Input: part model. Units: mm. Frame: model coordinates. Face numbers are marked on the shaded views. A direction names the side the tool comes from. Round coordinates to 2 decimals unless told otherwise and drop trailing zeros. Loops run counter-clockwise (first coordinate to the right, second up) from the corner with the lowest first, then second, coordinate; pieces in that order, holes last.
1) Access query for the marked faces 4 and 5. Directions: +Z, -Z, +X, -X, +Y, -Y. A direction counts if a zero-diameter tool reaches every point of the face in a straight line with its end or side. Return the directions, or none.
2) Draft query along Y for the marked faces 1, 2 and 3. Return one class per face: pulls with the +Y half, pulls with the -Y half, needs draft (parallel to the pull), parting line crosses it, or undercut.
3) Section A-A, the plane x = 0. Return loops of the section in (y, z), and give its area (3 significant figures).
4) Section D-D, the plane z = 4.5. Return loops of the section in (x, y).
5) Ray query, line 1 along Z through (x, y) = (4.75, 1.5); line 2 along Y through (x, z) = (0, 6.75); line 3 along X through (y, z) = (1.25, 7). Return the intervals inside material, ascending.
6) Section C-C, the plane y = -2.5. Return loops of the section in (x, z).
7) First-contact query: pin 1 (3 mm diameter, centred on x = -1.5, z = 3.5, fed in from -Y); pin 2 (1.5 mm diameter, centred on x = -3.5, z = 4.5, fed in from -Y); pin 3 (1.5 mm diameter, centred on x = -3.5, z = 2.5, fed in from +Y); pin 4 (1.8 mm diameter, centred on x = 0, y = 0, fed in from -Z). Flat tips, straight axial feed; report the tip coordinate or a pass-through.
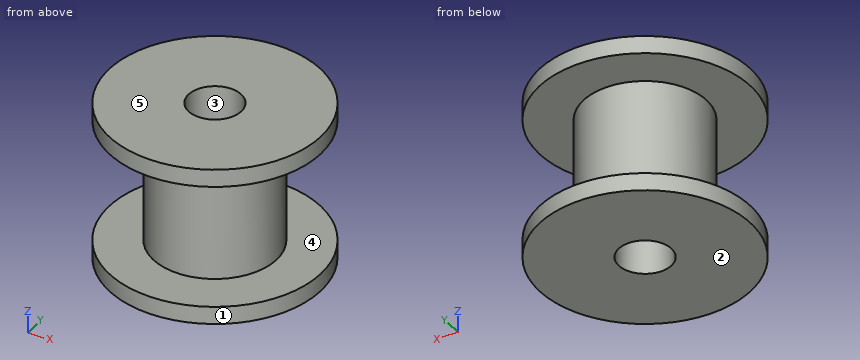
from build123d import *

# Parameters (mm, degrees)
SKETCH2_R               = 6
SKETCH2_R_2             = 1.5
BOSS_EXTRUDE1_DEPTH     = 9
CUT_EXTRUDE_THIN1_START = 1
SKETCH2_3_R             = 13.5
SKETCH2_3_R_2           = 3.5
CUT_EXTRUDE_THIN1_DEPTH = 7


with BuildPart() as part:
    # Sketch2 → Boss-Extrude1 (new body)
    with BuildSketch(Plane.XY):
        Circle(SKETCH2_R)
        Circle(SKETCH2_R_2, mode=Mode.SUBTRACT)
    extrude(amount=BOSS_EXTRUDE1_DEPTH)

    # Sketch2<3> → Cut-Extrude-Thin1 (cut)
    with BuildSketch(Plane.XY.offset(CUT_EXTRUDE_THIN1_START)):
        Circle(SKETCH2_3_R)
        Circle(SKETCH2_3_R_2, mode=Mode.SUBTRACT)
    extrude(amount=CUT_EXTRUDE_THIN1_DEPTH, mode=Mode.SUBTRACT)


solid = part.part
Final values:
1. face 4: none
1. face 5: +Z, +X, -X, +Y, -Y
2. face 1: parting line crosses it
2. face 2: needs draft
2. face 3: undercut
3. outline: (-6, 0) - (-1.5, 0) - (-1.5, 9) - (-6, 9) - (-6, 8) - (-3.5, 8) - (-3.5, 1) - (-6, 1) - close; (1.5, 0) - (6, 0) - (6, 1) - (3.5, 1) - (3.5, 8) - (6, 8) - (6, 9) - (1.5, 9) - close
3. area: 46.0 mm2
4. outline: circle Ø7 at (0, 0); hole circle Ø3 at (0, 0)
5. line 1: z = 0 to 1, 8 to 9
5. line 2: y = -3.5 to -1.5, 1.5 to 3.5
5. line 3: x = -3.27 to -0.83, 0.83 to 3.27
6. outline: (-5.45, 0) - (5.45, 0) - (5.45, 1) - (2.45, 1) - (2.45, 8) - (5.45, 8) - (5.45, 9) - (-5.45, 9) - (-5.45, 8) - (-2.45, 8) - (-2.45, 1) - (-5.45, 1) - close
7. pin 1: stops at y = -3.5
7. pin 2: stops at y = -2.17
7. pin 3: stops at y = 2.17
7. pin 4: passes through
